Build history of the part. All positions in model axes, mm. Face numbers are marked on the shaded views. A direction names the side the tool comes from. Round coordinates to 2 decimals unless told otherwise and drop trailing zeros. Write each loop counter-clockwise with the first axis right and the second up, starting at its lowest first coordinate (ties: lowest second). Pieces come first, ordered by that corner, then holes.
1) Saw through at C-C (y = 16.5). Write the cut outline in (x, z), plus the area to 3 significant figures.
2) Pull direction X, two halves, no side cores. Call the marked faces 4, 5 and 6: +X half, -X half, draft (parallel to the pull), parting line (faces both ways), or undercut.
3) Flat gauge pins, fed straight in: pin 1 (2 mm diameter, centred on x = -14, z = 5, fed in from +Y); pin 2 (2 mm diameter, centred on x = 6.5, z = 5, fed in from +Y); pin 3 (1.6 mm diameter, centred on x = 6.11, z = 5, fed in from +Y). Where does each tip first touch, or does it go through?
4) Which spindle directions (+Z, -Z, +X, -X, +Y, -Y) get a long thin tool onto all of the face, cutting with end or side? Do the marked faces 1, 2 and 3. Say none if no direction does.
5) Saw through at B-B (z = 5). Write the cut outline in (x, y).
6) Saw through at D-D (y = -1). Write the cut outline in (x, z).
7) Wall check: probe 1 along X at (y, z) = (13.25, 5); probe 2 along Z at (x, y) = (-13.75, 9.5); probe 3 along X at (y, z) = (5.15, 5). Give the ranges that are in metal, low to high.
8) Saw through at A-A (y = 6). Write the cut outline in (x, z).
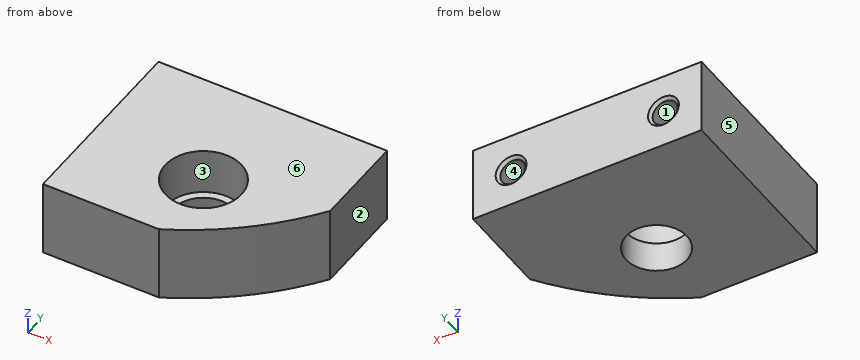
from build123d import *

# Parameters (mm, degrees)
SKIZZE1_W                       = 30
SKIZZE1_H                       = 25
SKIZZE1_R                       = 4
AUFSATZ_LINEAR_AUSTRAGEN1_DEPTH = 10
SKIZZE2_R                       = 5
SCHNITT_LINEAR_AUSTRAGEN1_DEPTH = 6
SKIZZE3_R                       = 1
SCHNITT_LINEAR_AUSTRAGEN2_DEPTH = 16
M4_GEWINDEBOHRUNG1_D            = 3.3
M4_GEWINDEBOHRUNG1_DEPTH        = 11.5
M4_GEWINDEBOHRUNG1_CSINK_D      = 4.05
M4_GEWINDEBOHRUNG1_CSINK_ANGLE  = 90
M4_GEWINDEBOHRUNG1_TIP          = 0.991420021
SKIZZE5_R                       = 51.207337477
SKIZZE5_R_2                     = 39
SCHNITT_LINEAR_AUSTRAGEN3_DEPTH = 10


with BuildPart() as part:
    # Skizze1 → Aufsatz-Linear austragen1 (new body)
    with BuildSketch(Plane.XY):
        with Locations((-3.885739266, 7.64084507)):
            Rectangle(SKIZZE1_W, SKIZZE1_H)
        with Locations((-3.885739266, 5.14084507)):
            Circle(SKIZZE1_R, mode=Mode.SUBTRACT)
    extrude(amount=AUFSATZ_LINEAR_AUSTRAGEN1_DEPTH)

    # Skizze2 → Schnitt-Linear austragen1 (cut)
    with BuildSketch(Plane.XY.offset(10)):
        with Locations((-3.885739266, 5.14084507)):
            Circle(SKIZZE2_R)
    extrude(amount=-SCHNITT_LINEAR_AUSTRAGEN1_DEPTH, mode=Mode.SUBTRACT)

    # Skizze3 → Schnitt-Linear austragen2 (cut)
    with BuildSketch(Plane(origin=(0, 20.14084507, 0), x_dir=(1, 0, 0), z_dir=(0, 1, 0))):
        with Locations(Location((-13.885739266, -5, 0), (0, 0, 270))):
            Circle(SKIZZE3_R)
        with Locations(Location((6.114260734, -5, 0), (0, 0, 270))):
            Circle(SKIZZE3_R)
    extrude(amount=-SCHNITT_LINEAR_AUSTRAGEN2_DEPTH, mode=Mode.SUBTRACT)

    # M4 Gewindebohrung1
    with Locations(Plane(origin=(-13.885739266, 20.14084507, 5), x_dir=(0, 0, 1), z_dir=(0, 1, 0))):
        with Locations((0, 0), (0, 20)):
            CounterSinkHole(M4_GEWINDEBOHRUNG1_D / 2, M4_GEWINDEBOHRUNG1_CSINK_D / 2, depth=M4_GEWINDEBOHRUNG1_DEPTH, counter_sink_angle=M4_GEWINDEBOHRUNG1_CSINK_ANGLE)
            with Locations((0, 0, -(M4_GEWINDEBOHRUNG1_DEPTH + M4_GEWINDEBOHRUNG1_TIP / 2))):  # 118° drill point
                Cone(0, M4_GEWINDEBOHRUNG1_D / 2, M4_GEWINDEBOHRUNG1_TIP, mode=Mode.SUBTRACT)

    # Skizze5 → Schnitt-Linear austragen3 (cut)
    with BuildSketch(Plane.XY.offset(10)):
        with Locations((-20.885739266, 30.14084507)):
            Circle(SKIZZE5_R)
        with Locations((-20.885739266, 30.14084507)):
            Circle(SKIZZE5_R_2, mode=Mode.SUBTRACT)
    extrude(amount=-SCHNITT_LINEAR_AUSTRAGEN3_DEPTH, mode=Mode.SUBTRACT)


solid = part.part
Evaluation:
1. outline: (-18.89, 0) - (11.11, 0) - (11.11, 10) - (-18.89, 10) - close; hole circle Ø3.3 at (-13.89, 5); hole circle Ø3.3 at (6.11, 5)
1. area: 283 mm2
2. face 4: undercut
2. face 5: -X half
2. face 6: draft
3. pin 1: stops at y = 8.32
3. pin 2: stops at y = 8.48
3. pin 3: stops at y = 4.14
4. face 1: +Y
4. face 2: +Z, -Z, +X, +Y, -Y
4. face 3: +Z
5. outline: (-18.89, -4.86) - (-3.68, -4.86) arc R39 ccw to (11.11, 7.85) - (11.11, 20.14) - (8.14, 20.14) - (7.76, 19.77) - (7.76, 8.64) - (7.11, 8.25) - (7.11, 4.14) - (5.11, 4.14) - (5.11, 8.25) - (4.46, 8.64) - (4.46, 19.77) - (4.09, 20.14) - (-11.86, 20.14) - (-12.24, 19.77) - (-12.24, 8.64) - (-12.89, 8.25) - (-12.89, 4.14) - (-14.89, 4.14) - (-14.89, 8.25) - (-15.54, 8.64) - (-15.54, 19.77) - (-15.91, 20.14) - (-18.89, 20.14) - close; hole circle Ø10 at (-3.89, 5.14)
6. outline: (-18.89, 0) - (2.59, 0) - (2.59, 10) - (-18.89, 10) - close
7. probe 1: x = -18.89 to -15.54, -12.24 to 4.46, 7.76 to 11.11
7. probe 2: z = 0 to 3.36, 6.64 to 10
7. probe 3: x = -18.89 to -14.89, -12.89 to -8.89, 1.11 to 5.11, 7.11 to 9.06
8. outline: (-18.89, 0) - (-7.79, 0) - (-7.79, 4) - (-8.81, 4) - (-8.81, 10) - (-18.89, 10) - close; (0.02, 0) - (9.74, 0) - (9.74, 10) - (1.04, 10) - (1.04, 4) - (0.02, 4) - close; hole circle Ø2 at (-13.89, 5); hole circle Ø2 at (6.11, 5)
